from build123d import *

# Parameters (mm, degrees)
SKETCH1_R           = 0.75
BOSS_EXTRUDE1_DEPTH = 5.1
SKETCH8_R           = 0.75
BOSS_EXTRUDE2_DEPTH = 1.75
SKETCH9_R           = 0.75
BOSS_EXTRUDE3_DEPTH = 8
SKETCH10_R          = 0.6
CUT_EXTRUDE7_DEPTH  = 5.65
SKETCH11_R          = 0.5
CUT_EXTRUDE8_DEPTH  = 6.5
CUT_EXTRUDE9_DEPTH  = 14.85
CUT_EXTRUDE10_DEPTH = 6.5
FILLET2_R           = 0.15
CUT_EXTRUDE11_DEPTH = 2.2
FILLET3_R           = 0.4
SKETCH17_R          = 0.75
SKETCH16_R          = 0.8


with BuildPart() as part:
    # Sketch1 → Boss-Extrude1 (new body)
    with BuildSketch(Plane.XY):
        Circle(SKETCH1_R)
    extrude(amount=BOSS_EXTRUDE1_DEPTH)

    # Sketch8 → Boss-Extrude2 (add)
    with BuildSketch(Plane.XY.offset(5.1)):
        Circle(SKETCH8_R)
    extrude(amount=BOSS_EXTRUDE2_DEPTH)

    # Sketch9 → Boss-Extrude3 (add)
    with BuildSketch(Plane.XY.offset(6.85)):
        Circle(SKETCH9_R)
    extrude(amount=BOSS_EXTRUDE3_DEPTH)

    # Sketch10 → Cut-Extrude7 (cut)
    with BuildSketch(Plane.XY.offset(14.85)):
        Circle(SKETCH10_R)
    extrude(amount=-CUT_EXTRUDE7_DEPTH, mode=Mode.SUBTRACT)

    # Sketch11 → Cut-Extrude8 (cut)
    with BuildSketch(Plane(origin=(0, 0, 0), x_dir=(-1, 0, 0), z_dir=(0, 0, -1))):
        Circle(SKETCH11_R)
    extrude(amount=-CUT_EXTRUDE8_DEPTH, mode=Mode.SUBTRACT)

    # Sketch12 → Cut-Extrude9 (cut)
    with BuildSketch(Plane.XY.offset(14.85)):
        with BuildLine():
            Line((-0.03, 0.74939976), (-0.03, 0.599249531))
            ThreePointArc((-0.03, 0.599249531), (0, 0.6), (0.03, 0.599249531))
            Line((0.03, 0.599249531), (0.03, 0.74939976))
            ThreePointArc((0.03, 0.74939976), (0, 0.75), (-0.03, 0.74939976))
        make_face()
    extrude(amount=-CUT_EXTRUDE9_DEPTH, mode=Mode.SUBTRACT)

    # Sketch14 → Cut-Extrude10 (cut)
    with BuildSketch(Plane(origin=(0, 0, 0), x_dir=(-1, 0, 0), z_dir=(0, 0, -1))):
        with BuildLine():
            Line((-0.03, 0.74939976), (-0.03, 0.499099189))
            ThreePointArc((-0.03, 0.499099189), (0, 0.5), (0.03, 0.499099189))
            Line((0.03, 0.499099189), (0.03, 0.74939976))
            ThreePointArc((0.03, 0.74939976), (0, 0.75), (-0.03, 0.74939976))
        make_face()
    extrude(amount=-CUT_EXTRUDE10_DEPTH, mode=Mode.SUBTRACT)

    # Fillet2
    fillet2_edges = [part.edges().sort_by_distance(p)[0] for p in [
        (0.34278273, -0.364005494, 0),
    ]]
    fillet(fillet2_edges, radius=FILLET2_R)

    # Sketch15 → Cut-Extrude11 (cut)
    with BuildSketch(Plane.XY.offset(14.85)):
        with BuildLine():
            Line((-0.749733286, -0.02), (-0.599666574, -0.02))
            ThreePointArc((-0.599666574, -0.02), (-0.441573883, 0.406217314), (-0.03, 0.599249531))
            Line((-0.03, 0.599249531), (-0.03, 0.74939976))
            ThreePointArc((-0.03, 0.74939976), (-0.547713426, 0.5123573), (-0.749733286, -0.02))
        make_face()
        with BuildLine():
            Line((0.03, 0.599249531), (0.03, 0.74939976))
            ThreePointArc((0.03, 0.74939976), (0.547713426, 0.5123573), (0.749733286, -0.02))
            Line((0.749733286, -0.02), (0.599666574, -0.02))
            ThreePointArc((0.599666574, -0.02), (0.441573883, 0.406217314), (0.03, 0.599249531))
        make_face()
    extrude(amount=-CUT_EXTRUDE11_DEPTH, mode=Mode.SUBTRACT)

    # Fillet3
    fillet3_edges = [part.edges().sort_by_distance(p)[0] for p in [
        (-0.67469993, -0.02, 12.65),
        (-0.67469993, -0.02, 14.85),
        (0.67469993, -0.02, 12.65),
        (0.67469993, -0.02, 14.85),
    ]]
    fillet(fillet3_edges, radius=FILLET3_R)

    # Sketch17 → Loft1 section 0
    with BuildSketch(Plane.XY.offset(8.35)):
        Circle(SKETCH17_R)
    # Sketch16 → Loft1 section 1
    with BuildSketch(Plane.XY.offset(8.85)):
        Circle(SKETCH16_R)
    loft()


solid = part.part
Geometry check sheet. Reference: the model listing, model coordinates, mm. A direction names the side the tool comes from. Round coordinates to 2 decimals unless told otherwise and drop trailing zeros. Order: outer loops, then holes, each group sorted by start corner. A loop starts at its lowest first (then second) coordinate and runs counter-clockwise, first axis right, second up. Notation, with made-up numbers: (39.5, 75.25) - (51.5, 75.25) arc R18 cw to (51.5, 93.25) - close; hole circle Ø2 at (-6, -1.5). An arc over 180 degrees is marked (long way). One line per question, with ' | ' between items. Start each with the question number.
(1) Access from +Z, -Z, +X, -X, +Y, -Y to the whole of each face (thin tool, end or side, straight path). Record for faces 1 (the cylindrical face through (-0.03, -0.75, 11.14)), 2 (the flat face through (0, 0, 6.5)).
(2) Thickness scan on L1, parallel to X at y = 0, z = 5; L2, parallel to X at y = -0.05, z = 11; L3, parallel to Z at x = -0.3, y = -0.25. Record the ranges inside material, lowest first. Write a range as [from, to].
(3) Release check for a two-part mould opening along Y. For faces 3 (the cylindrical face through (0, -0.6, 11.4)), 4 (the flat face through (0, 0, 9.2)), 5 (the cylindrical face through (-0.03, -0.75, 4.12)) record: released by +Y, released by -Y, zero draft, split by the parting line, or undercut.
(4) Sectioned sample at A-A on z = 4.75. Record the cut outline in (x, y), and give its area (3 significant figures).
(5) Sectioned sample at B-B on z = 9. Record the cut outline in (x, y).
(6) Depth check by flat-ended pin: pin 1 Ø0.8 at (x, y) = (0, 0) entering from -Z. Enter the tip coordinate at first touch or a pass-through.
Conclusion:
1) face 1: +Z | face 2: -Z
2) L1: x = [-0.75, -0.5], [0.5, 0.75] | L2: x = [-0.75, -0.6], [0.6, 0.75] | L3: z = [6.5, 9.2]
3) face 3: undercut | face 4: undercut | face 5: split by the parting line
4) outline: (-0.03, 0.5) - (-0.03, 0.75) arc R0.75 ccw (long way) to (0.03, 0.75) - (0.03, 0.5) arc R0.5 cw (long way) to start | area: 0.967 mm2
5) outline: (-0.03, 0.6) - (-0.03, 0.75) arc R0.75 ccw (long way) to (0.03, 0.75) - (0.03, 0.6) arc R0.6 ccw to start
6) pin 1: stops at z = 6.5
